Autodesk Inventor part; units mm, degrees
ref_plane "YZ Plane" through (0, 0, 0) normal (1, 0, 0) x (0, 1, 0)
ref_plane "XZ Plane" through (0, 0, 0) normal (0, 1, 0) x (-1, 0, 0)
ref_plane "XY Plane" through (0, 0, 0) normal (0, 0, 1) x (1, 0, 0)
sketch "草圖1" plane through (0, 0, 0) normal (0, 1, 0) x (-1, 0, 0)
  line L0 (0, 0) -> (0, -140)
  line L1 (15, -140) -> (15, 0)
  line L2 (3.35, 0) -> (3.35, 3)
  line L3 (3.35, 3) -> (11.65, 3)
  line L4 (11.65, 3) -> (11.65, 0)
  line L5 (3.35, -140) -> (3.35, -143)
  line L6 (3.35, -143) -> (11.65, -143)
  line L7 (11.65, -143) -> (11.65, -140)
  line L8 (0, -140) -> (3.35, -140)
  line L9 (11.65, -140) -> (15, -140)
  line L10 (15, 0) -> (11.65, 0)
  line L11 (3.35, 0) -> (0, 0)
  dimension "d0" = 3
  dimension "d1" = 8.3
  dimension "d2" = 15
  dimension "d4" = 3
  dimension "d5" = 8.3
  dimension "d7" = 140
  dimension "d8" = 140
  dimension "d28" = 3.35
  dimension "d29" = 3.35
extrude "擠出1" add sketch "草圖1" along normal blind 3
sketch "草圖3" plane through (0, 0, 0) normal (0, -1, 0) x (1, 0, 0)
  line L0 (5, 3) -> (0, 3)
  line L1 (0, 3) -> (0, -143)
  line L2 (0, -143) -> (5, -143)
  line L3 (5, -143) -> (5, 3)
  line L4 (0, 0) -> (0, -140)
  line L5 (-11.65, 3) -> (-3.35, 3)
  dimension "d24" = 146
  dimension "d25" = 5
extrude "擠出3" [suppressed]
sketch "草圖2" plane through (0, 3, 0) normal (0, 1, 0) x (1, 0, 0)
  line L0 (0, 140) -> (-3.35, 140)
  line L1 (-3.35, 140) -> (-3.35, 143)
  line L2 (-3.35, 143) -> (-11.65, 143)
  line L3 (-11.65, 143) -> (-11.65, 140)
  line L4 (-11.65, 140) -> (-15, 140)
  line L5 (-15, 140) -> (-15, 0)
  line L6 (-15, 0) -> (-11.65, 0)
  line L7 (-11.65, 0) -> (-11.65, -3)
  line L8 (-11.65, -3) -> (-3.35, -3)
  line L9 (-3.35, -3) -> (-3.35, 0)
  line L10 (-3.35, 0) -> (0, 0)
  line L11 (-4, 134) -> (1, 134)
  line L12 (1, 134) -> (1, 6)
  line L13 (1, 6) -> (-4, 6)
  line L14 (-4, 6) -> (-4, 134)
  line L15 (-4, 67.5707) -> (-4, 72.4293)
  line L16 (-5, 72.4293) -> (-5, 67.5707)
  line L17 (5, 143) -> (5, -3)
  line L18 (0, 0) -> (0, 140)
  dimension "d17" = 5
  dimension "d19" = 6
  dimension "d20" = 6
  dimension "d30" = 4
extrude "擠出2" [suppressed]
sketch "草圖4" plane through (0, 3, 0) normal (0, 1, 0) x (1, 0, 0)
  line L0 (0, 0) -> (0, 140)
  line L1 (0, 140) -> (-3.35, 140)
  line L2 (-3.35, 140) -> (-3.35, 143)
  line L3 (-3.35, 143) -> (-11.65, 143)
  line L4 (-11.65, 143) -> (-11.65, 140)
  line L5 (-11.65, 140) -> (-15, 140)
  line L6 (-15, 140) -> (-15, 0)
  line L7 (-15, 0) -> (-11.65, 0)
  line L8 (-11.65, 0) -> (-11.65, -3)
  line L9 (-11.65, -3) -> (-3.35, -3)
  line L10 (-3.35, -3) -> (-3.35, 0)
  line L11 (-3.35, 0) -> (0, 0)
equation "\"d29\" = d28"
properties part number "chassis_1_3"
Can you work these out from the model? Positions are in its coordinate system, mm. A direction names the side the tool comes from. Coordinates: 2 decimals unless noted, no trailing zeros. Write each loop counter-clockwise with the first axis right and the second up, starting at its lowest first coordinate (ties: lowest second). Pieces come first, ordered by that corner, then holes. Notation, with made-up numbers: M 30.5,15.5 L 81.5,15.5 A11 cw 81.5,27.5 Z; hole C -27,57 d1. An arc over 180 degrees is marked long. Use one line per item in the form item = value.
Q1. If we section it at B-B (x = -1.25): Write out the boundary of the cut face in (y, z), then the cut area to 3 significant figures.
Model answer:
outline = M 0,-140 L 3,-140 L 3,0 L 0,0 Z
area = 420 mm^2
Q2. For faces 1 (the flat face through (-13, 1, -140)), 2 (the flat face through (-3.35, 1, 1)), 3 (the flat face through (-3.35, 1, -141)), 4 (the flat face through (-13, 1, 0)), 5 (the flat face through (-15, 1, -71)), which set-ups out of +Z, -Z, +X, -X, +Y, -Y let a thin tool reach every point of the face, with its end or its side?
Model answer:
face_1 = -Z, -X, +Y, -Y
face_2 = +Z, +X, +Y, -Y
face_3 = -Z, +X, +Y, -Y
face_4 = +Z, -X, +Y, -Y
face_5 = +Z, -Z, -X, +Y, -Y
Q3. If we section it at A-A (y = 2.55): Write out the boundary of the cut face in (x, z).
Model answer:
outline = M -15,-140 L -11.65,-140 L -11.65,-143 L -3.35,-143 L -3.35,-140 L 0,-140 L 0,0 L -3.35,0 L -3.35,3 L -11.65,3 L -11.65,0 L -15,0 Z
Q4. For P1, Ø2, axis at x = -4.5, z = -104, coming from the -Y side; P2, Ø1.5, axis at x = -13.5, y = 1, coming from the -Z side; P3, Ø1.5, axis at x = -2.5, y = 0.5, coming from the +Z side; P4, Ø1.5, axis at y = 1.5, z = -142, coming from the +X side, each with a flat end and sliding along its axis, tell me the tip position at first contact or that it passes through.
Model answer:
P1 = 0
P2 = -140
P3 = 0
P4 = -3.35
Q5. I need wall thicknesses on line 1 along Z through (x, y) = (-2.75, 2.4). Which ranges of the line are inside material? Lowest first, please. Write a range as from..to.
Model answer:
line_1 = -140..0
